Work out the finished part from the listing and answer in its coordinate system (mm). A direction names the side the tool comes from. Give positions to 0.01 mm unless a question says otherwise; leave off trailing zeros. Order: outer loops, then holes, each group sorted by start corner. A loop starts at its lowest first (then second) coordinate and runs counter-clockwise, first axis right, second up. Notation, with made-up numbers: (43.5, 2) - (89.5, 2) arc R8 cw to (89.5, 16) - close; hole circle Ø6 at (18.25, -29.75). An arc over 180 degrees is marked (long way). Put each result on its own line as item: value.
```python
from build123d import *

# Parameters (mm, degrees)
AUFSATZ_LINEAR_AUSTRAGEN1_DEPTH        = 6
SKIZZE2_W                              = 6
SKIZZE2_H                              = 20
AUFSATZ_LINEAR_AUSTRAGEN2_DEPTH        = 7.9
SKIZZE3_W                              = 6
SKIZZE3_H                              = 20
AUFSATZ_LINEAR_AUSTRAGEN3_DEPTH        = 7.9
SKIZZE4_R                              = 7.15
AUFSATZ_LINEAR_AUSTRAGEN4_DEPTH        = 7
SKIZZE5_W                              = 19
SKIZZE5_H                              = 19
SCHNITT_LINEAR_AUSTRAGEN1_DEPTH        = 1.3
SKIZZE6_W                              = 18
SKIZZE6_H                              = 18
SCHNITT_LINEAR_AUSTRAGEN2_DEPTH        = 3.7
F_1_5_1_5_DURCHMESSER_BOHRUNG1_D       = 1.5
F_1_5_1_5_DURCHMESSER_BOHRUNG1_DEPTH   = 13
F_10_8_10_8_DURCHMESSER_BOHRUNG1_D     = 10.8
F_10_8_10_8_DURCHMESSER_BOHRUNG1_DEPTH = 13
F_1_6_1_6_DURCHMESSER_BOHRUNG1_REACH   = 25.785
F_1_6_1_6_DURCHMESSER_BOHRUNG1_BORE_R  = 0.8
FASE1_SIZE                             = 2
FASE2_SIZE                             = 2.292893219


with BuildPart() as part:
    # Skizze1 → Aufsatz-Linear austragen1 (new body)
    with BuildSketch(Plane(origin=(0, 0, 0), x_dir=(-1, 0, 0), z_dir=(0, 0, -1))):
        with BuildLine():
            Line((2.1, -11), (2.1, 11))
            ThreePointArc((2.1, 11), (0, 13.1), (-2.1, 11))
            Line((-2.1, 11), (-2.1, -11))
            ThreePointArc((-2.1, -11), (0, -13.1), (2.1, -11))
        make_face()
    extrude(amount=-AUFSATZ_LINEAR_AUSTRAGEN1_DEPTH)

    # Skizze2 → Aufsatz-Linear austragen2 (add)
    with BuildSketch(Plane.ZY.offset(2.1)):
        with Locations((3, 0)):
            Rectangle(SKIZZE2_W, SKIZZE2_H)
    extrude(amount=AUFSATZ_LINEAR_AUSTRAGEN2_DEPTH)

    # Skizze3 → Aufsatz-Linear austragen3 (add)
    with BuildSketch(Plane(origin=(2.1, 0, 0), x_dir=(0, 0, -1), z_dir=(1, 0, 0))):
        with Locations((-3, 0)):
            Rectangle(SKIZZE3_W, SKIZZE3_H)
    extrude(amount=AUFSATZ_LINEAR_AUSTRAGEN3_DEPTH)

    # Skizze4 → Aufsatz-Linear austragen4 (add)
    with BuildSketch(Plane.XY.offset(6)):
        with Locations(Location((0, 0, 0), (0, 0, 180))):
            Circle(SKIZZE4_R)
    extrude(amount=AUFSATZ_LINEAR_AUSTRAGEN4_DEPTH)

    # Skizze5 → Schnitt-Linear austragen1 (cut)
    with BuildSketch(Plane(origin=(0, 0, 0), x_dir=(-1, 0, 0), z_dir=(0, 0, -1))):
        Rectangle(SKIZZE5_W, SKIZZE5_H)
    extrude(amount=-SCHNITT_LINEAR_AUSTRAGEN1_DEPTH, mode=Mode.SUBTRACT)

    # Skizze6 → Schnitt-Linear austragen2 (cut)
    with BuildSketch(Plane(origin=(0, 0, 1.3), x_dir=(-1, 0, 0), z_dir=(0, 0, -1))):
        Rectangle(SKIZZE6_W, SKIZZE6_H)
    extrude(amount=-SCHNITT_LINEAR_AUSTRAGEN2_DEPTH, mode=Mode.SUBTRACT)

    # Ø1.5 (1.5) Durchmesser Bohrung1
    with Locations(Plane(origin=(0, 0, 0), x_dir=(-1, 0, 0), z_dir=(0, 0, -1))):
        with Locations((0, -11), (0, 11)):
            Hole(F_1_5_1_5_DURCHMESSER_BOHRUNG1_D / 2, depth=F_1_5_1_5_DURCHMESSER_BOHRUNG1_DEPTH)

    # Ø10.8 (10.8) Durchmesser Bohrung1
    with Locations(Plane.XY.offset(13)):
        with Locations((0, 0)):
            Hole(F_10_8_10_8_DURCHMESSER_BOHRUNG1_D / 2, depth=F_10_8_10_8_DURCHMESSER_BOHRUNG1_DEPTH)

    # Ø1.6 (1.6) Durchmesser Bohrung1 bore (on position points) → Ø1.6 (1.6) Durchmesser Bohrung1 (cut, up to next)
    with BuildSketch(Plane(origin=(7.15, 0, 10), x_dir=(0, 1, 0), z_dir=(1, 0, 0)), mode=Mode.PRIVATE) as f_1_6_1_6_durchmesser_bohrung1_sk1:
        Circle(F_1_6_1_6_DURCHMESSER_BOHRUNG1_BORE_R)
    f_1_6_1_6_durchmesser_bohrung1_tool1 = extrude(f_1_6_1_6_durchmesser_bohrung1_sk1.sketch, amount=-F_1_6_1_6_DURCHMESSER_BOHRUNG1_REACH, mode=Mode.PRIVATE) & part.part
    add(f_1_6_1_6_durchmesser_bohrung1_tool1.solids().sort_by_distance((7.15, 0, 10))[0], mode=Mode.SUBTRACT)

    # Fase1
    fase1_edges = [part.edges().sort_by_distance(p)[0] for p in [
        (-9, -9, 3.15),
        (9, -9, 3.15),
        (9, 9, 3.15),
        (-9, 9, 3.15),
    ]]
    chamfer(fase1_edges, length=FASE1_SIZE)

    # Fase2
    fase2_edges = [part.edges().sort_by_distance(p)[0] for p in [
        (9.5, 9.5, 0.65),
        (-9.5, 9.5, 0.65),
        (-9.5, -9.5, 0.65),
        (9.5, -9.5, 0.65),
    ]]
    chamfer(fase2_edges, length=FASE2_SIZE)


solid = part.part
```
(1) Straight lines are drawn through the part: line 1 (Y direction, x = 0, z = 4.15); line 2 (X direction, y = 6.75, z = 3.5). For each, find the intervals that lie inside material, in ascending order.
Geometry check:
line 1: y = -13.1 to -11.75, -10.25 to -9, 9 to 10.25, 11.75 to 13.1
line 2: x = -10 to -9, 9 to 10
(2) Section B-B, the plane y = -2.25 is taken. Write down the section's boundary in (x, z).
Geometry check:
outline: (-10, 0) - (-9.5, 0) - (-9.5, 1.3) - (-9, 1.3) - (-9, 5) - (-4.91, 5) - (-4.91, 13) - (-6.79, 13) - (-6.79, 6) - (-10, 6) - close; (4.91, 5) - (9, 5) - (9, 1.3) - (9.5, 1.3) - (9.5, 0) - (10, 0) - (10, 6) - (6.79, 6) - (6.79, 13) - (4.91, 13) - close
(3) Given pin 1 (2.5 mm diameter, centred on y = 0, z = 10, fed in from +X); pin 2 (6.5 mm diameter, centred on x = -7.5, z = 4, fed in from -Y); pin 3 (6.5 mm diameter, centred on x = 5, z = 3, fed in from +Y), each flat-ended and moving along its own axis, determine where each tip first touches the part or whether it passes through.
Geometry check:
pin 1: stops at x = 7.15
pin 2: stops at y = -10
pin 3: stops at y = 12.16
(4) Section C-C, the plane z = 1 is taken. Write down the section's boundary in (x, y), then the cut area to 3 significant figures.
Geometry check:
outline: (-10, -10) - (-2.1, -10) - (-2.1, -11) arc R2.1 ccw to (2.1, -11) - (2.1, -10) - (10, -10) - (10, 10) - (2.1, 10) - (2.1, 11) arc R2.1 ccw to (-2.1, 11) - (-2.1, 10) - (-10, 10) - close; hole (-9.5, -7.21) - (-7.21, -9.5) - (7.21, -9.5) - (9.5, -7.21) - (9.5, 7.21) - (7.21, 9.5) - (-7.21, 9.5) - (-9.5, 7.21) - close; hole circle Ø1.5 at (0, -11); hole circle Ø1.5 at (0, 11)
area: 68.2 mm²
(5) Section A-A, the plane x = 0 is taken. Write down the section's boundary in (y, z), then the cut area to 3 significant figures.
Geometry check:
outline: (-13.1, 0) - (-11.75, 0) - (-11.75, 6) - (-13.1, 6) - close; (-10.25, 0) - (-9.5, 0) - (-9.5, 1.3) - (-9, 1.3) - (-9, 5) - (-5.4, 5) - (-5.4, 13) - (-7.15, 13) - (-7.15, 6) - (-10.25, 6) - close; (5.4, 5) - (9, 5) - (9, 1.3) - (9.5, 1.3) - (9.5, 0) - (10.25, 0) - (10.25, 6) - (7.15, 6) - (7.15, 13) - (5.4, 13) - close; (11.75, 0) - (13.1, 0) - (13.1, 6) - (11.75, 6) - close
area: 61.6 mm²
(6) A tool of negligible diameter and unlimited length cuts with its end or side. For faces 1 (the face through (-4, -4, 5)), 2 (the face through (6.258, -0.104, 10.793)), 3 (the face through (-2.1, -10.5, 3)), 4 (the face through (6, 10, 3)), from which of +Z, -Z, +X, -X, +Y, -Y can it reach the whole face along a straight path? Write none if from no direction.
Geometry check:
face 1: -Z
face 2: +X
face 3: +Z, -Z, -X, -Y
face 4: +Z, -Z, +X, +Y
(7) Section D-D, the plane x = 3.25 is taken. Write down the section's boundary in (y, z).
Geometry check:
outline: (-10, 0) - (-9.5, 0) - (-9.5, 1.3) - (-9, 1.3) - (-9, 5) - (-4.31, 5) - (-4.31, 13) - (-6.37, 13) - (-6.37, 6) - (-10, 6) - close; (4.31, 5) - (9, 5) - (9, 1.3) - (9.5, 1.3) - (9.5, 0) - (10, 0) - (10, 6) - (6.37, 6) - (6.37, 13) - (4.31, 13) - close
(8) Determine the mould class of faces 5 (the face through (5, 6, 6)), 6 (the face through (-6, 10, 3)), 7 (the face through (0, -9, 3)) for opening direction Y: pulls with the +Y half, pulls with the -Y half, needs draft (parallel to the pull), parting line crosses it, or undercut.
Geometry check:
face 5: needs draft
face 6: pulls with the +Y half
face 7: undercut
